```python
from build123d import *

# Parameters (mm, degrees)
F1_DEPTH = 50.8
F3_D     = 22.86
F5_D     = 17.78
F7_DEPTH = 25.4


with BuildPart() as f1:
    # F0 (on Front) → F1 (new body, symmetric)
    with BuildSketch(Plane.XZ):
        with BuildLine():
            Line((-143.2661156607, -19.5504479766), (-143.2661156607, -44.9504479766))
            Line((-143.2661156607, -44.9504479766), (-79.7661156607, -44.9504479766))
            ThreePointArc((-79.7661156607, -44.9504479766), (-19.4636605074, -1.3467768462), (40.8387946459, -44.9504479766))
            Line((40.8387946459, -44.9504479766), (104.3387946459, -44.9504479766))
            Line((104.3387946459, -44.9504479766), (104.3387946459, -19.5504479766))
            Line((104.3387946459, -19.5504479766), (53.5387946459, -19.5504479766))
            ThreePointArc((53.5387946459, -19.5504479766), (-19.4636605074, 18.6164115569), (-92.4661156607, -19.5504479766))
            Line((-92.4661156607, -19.5504479766), (-143.2661156607, -19.5504479766))
        make_face()
    extrude(amount=F1_DEPTH, both=True)

    # F3 (through all)
    with Locations(Plane.XY.offset(-19.5504479766)):
        with Locations((-115.3261156607, 20.2373286647), (-115.3261156607, -25.4826713353)):
            Hole(F3_D / 2)

    # F5 (through all)
    with Locations(Plane.XY):
        with Locations((78.9387946459, 0)):
            Hole(F5_D / 2)

    # F6 (on face) → F7 (cut)
    with BuildSketch(Plane.XY.offset(-19.5504479766)):
        with BuildLine():
            ThreePointArc((87.8287946459, 0), (85.3648331771, -6.1431367229), (79.338776919, -8.8809973641))
            Line((79.338776919, -8.8809973641), (104.3387946459, -8.8809973641))
            Line((104.3387946459, -8.8809973641), (104.3387946459, 8.8899307883))
            Line((104.3387946459, 8.8899307883), (78.9738742688, 8.8899307883))
            ThreePointArc((78.9738742688, 8.8899307883), (85.2373642393, 6.273764506), (87.8287946459, 0))
        make_face()
    extrude(amount=-F7_DEPTH, mode=Mode.SUBTRACT)


solid = f1.part
```
Geometry check sheet. Reference: the model listing, model coordinates, mm. A direction names the side the tool comes from. Round coordinates to 2 decimals unless told otherwise and drop trailing zeros. Order: outer loops, then holes, each group sorted by start corner. A loop starts at its lowest first (then second) coordinate and runs counter-clockwise, first axis right, second up. Notation, with made-up numbers: (6, 15.5) -> (48, 15.5) arc R11 ccw to (48, 20.5) -> close; hole circle Ø10 at (6.5, -39). An arc over 180 degrees is marked (long way). Return JSON: item names as keys, results as strings. Group by question number.
Q1. Release check for a two-part mould opening along X. For faces 1 (the cylindrical face through (-125.885, -29.86, -32.428)), 2 (the flat face through (92, -8.881, -32)), 3 (the flat face through (104.339, -30, -32)) record: released by +X, released by -X, zero draft, split by the parting line, or undercut.
Q2. Material ranges on probe 1 along Y at (x, z) = (-124.5, -34.5); probe 2 along Z at (x, y) = (-97, -22.5); probe 3 along X at (y, z) = (26, -15), recorded low to high. Write a range as from..to.
Q3. Section check B-B, the plane x = -110.5. Record the boundary of the cut face in (y, z), plus the area to 3 significant figures.
Q4. Section check A-A, the plane y = 23.5. Record the boundary of the cut face in (x, z), plus the area to 3 significant figures.
Q5. Section check D-D, the plane z = 5. Record the boundary of the cut face in (x, y).
Q6. Section check C-C, the plane y = 0. Record the boundary of the cut face in (x, z).
Q7. Gauge pin test, flat ends, axial feed: pin 1 (1 mm diameter, centred on y = 14.5, z = -11.5, fed in from +X); pin 2 (3 mm diameter, centred on x = -29.5, y = -11.5, fed in from -Z); pin 3 (3 mm diameter, centred on y = -14, z = -5.5, fed in from -X). Record the tip position at first contact, or that the pin passes through.
Q8. Tool access check on faces 4 (the flat face through (68, -1, -19.55)), 5 (the flat face through (92, 8.89, -32)), 6 (the cylindrical face through (-126.23, 23.67, -32.43)), 7 (the flat face through (-118, -1, -19.55)), 8 (the flat face through (-21, -50.8, 1)). Record the directions out of +Z, -Z, +X, -X, +Y, -Y that give a thin tool (end or side, any length) a straight path to the whole face; none if there is none.
Numbers:
{
 "1": {"face 1": "undercut", "face 2": "zero draft", "face 3": "released by +X"},
 "2": {"probe 1": "-50.8..-32.3, -18.66..13.42, 27.06..50.8", "probe 2": "-44.95..-19.55", "probe 3": "-89.08..-58.8, 19.88..50.16"},
 "3": {"outline": "(-50.8, -44.95) -> (-35.84, -44.95) -> (-35.84, -19.55) -> (-50.8, -19.55) -> close; (-15.12, -44.95) -> (9.88, -44.95) -> (9.88, -19.55) -> (-15.12, -19.55) -> close; (30.6, -44.95) -> (50.8, -44.95) -> (50.8, -19.55) -> (30.6, -19.55) -> close", "area": "1,530 mm^2"},
 "4": {"outline": "(-143.27, -44.95) -> (-126.28, -44.95) -> (-126.28, -19.55) -> (-143.27, -19.55) -> close; (-104.37, -44.95) -> (-79.77, -44.95) arc R63.5 cw to (40.84, -44.95) -> (104.34, -44.95) -> (104.34, -19.55) -> (53.54, -19.55) arc R88.9 ccw to (-92.47, -19.55) -> (-104.37, -19.55) -> close", "area": "5,790 mm^2"},
 "5": {"outline": "(-66.75, -50.8) -> (27.82, -50.8) -> (27.82, 50.8) -> (-66.75, 50.8) -> close"},
 "6": {"outline": "(-143.27, -44.95) -> (-79.77, -44.95) arc R63.5 cw to (40.84, -44.95) -> (70.05, -44.95) -> (70.05, -19.55) -> (53.54, -19.55) arc R88.9 ccw to (-92.47, -19.55) -> (-143.27, -19.55) -> close"},
 "7": {"pin 1": "x = 47.66", "pin 2": "z = -2.4", "pin 3": "x = -81.9"},
 "8": {"face 4": "+Z, +X, +Y, -Y", "face 5": "+Z, -Z, +X", "face 6": "+Z, -Z", "face 7": "+Z, -X, +Y, -Y", "face 8": "+Z, -Z, +X, -X, -Y"}
}
